For this review, take the finished solid that the model builds, in its own axes (mm). A direction names the side the tool comes from. Coordinates: 2 decimals unless noted, no trailing zeros. Write each loop counter-clockwise with the first axis right and the second up, starting at its lowest first coordinate (ties: lowest second). Pieces come first, ordered by that corner, then holes.
```python
from build123d import *

# Parameters (mm, degrees)
ESBO_O1_R                  = 12.15
RESSALTO_EXTRUS_O1_DEPTH   = 15
ESBO_O2_R                  = 4.5
RESSALTO_EXTRUS_O2_DEPTH   = 15.5
ESBO_O3_R                  = 0.9
CORTE_EXTRUS_O1_DEPTH      = 19.5
CORTE_EXTRUS_O1_DEPTH_BACK = 15.5


with BuildPart() as part:
    # Esboço1 → Ressalto-extrusão1 (new body)
    with BuildSketch(Plane.XY):
        Circle(ESBO_O1_R)
    extrude(amount=RESSALTO_EXTRUS_O1_DEPTH)

    # Esboço2 → Ressalto-extrusão2 (add)
    with BuildSketch(Plane.XY):
        Circle(ESBO_O2_R)
    extrude(amount=RESSALTO_EXTRUS_O2_DEPTH)

    # Esboço3 → Corte-extrusão1 (cut, two sides)
    with BuildSketch(Plane.XY) as corte_extrus_o1_sk:
        Circle(ESBO_O3_R)
    extrude(amount=CORTE_EXTRUS_O1_DEPTH, mode=Mode.SUBTRACT)
    extrude(corte_extrus_o1_sk.sketch, amount=-CORTE_EXTRUS_O1_DEPTH_BACK, mode=Mode.SUBTRACT)


solid = part.part
```
Q1. Tool access review of faces 1 (the flat face through (-1.1, 0.1, 15.5)), 2 (the flat face through (5, 0, 15)): name each direction out of +Z, -Z, +X, -X, +Y, -Y from which nothing blocks a thin tool from reaching the whole face with its end or side.
Ans:
face 1: +Z, +X, -X, +Y, -Y
face 2: +Z
Q2. Draft analysis for pull direction X (two halves, no side actions). For faces 3 (the cylindrical face through (0.86, 0.27, 7.64)), 4 (the cylindrical face through (-2.63, -11.86, 7.4)), 5 (the flat face through (0, -3, 0)), state which applies: +X half, -X half, draft (parallel to the pull), parting line (faces both ways), or undercut.
Ans:
face 3: undercut
face 4: parting line
face 5: draft
Q3. Add section A-A (y = 0). State the section outline as (x, z) points.
Ans:
outline: (-12.15, 0) - (-0.9, 0) - (-0.9, 15.5) - (-4.5, 15.5) - (-4.5, 15) - (-12.15, 15) - close; (0.9, 0) - (12.15, 0) - (12.15, 15) - (4.5, 15) - (4.5, 15.5) - (0.9, 15.5) - close
Q4. For probe 1 along Y at (x, z) = (0, 6.5); probe 2 along Z at (x, y) = (-2.75, -7.5); probe 3 along Y at (x, z) = (-0.75, 1), list the stretches that pass through material, from the lowest coordinate up.
Ans:
probe 1: y = -12.15 to -0.9, 0.9 to 12.15
probe 2: z = 0 to 15
probe 3: y = -12.13 to -0.5, 0.5 to 12.13
Q5. Add section C-C (z = 7.25). State the section outline as (x, y) points.
Ans:
outline: circle Ø24.3 at (0, 0); hole circle Ø1.8 at (0, 0)
Q6. Clearance check with flat-ended pins moving along their axes: pin 1 Ø3 at (x, z) = (5.5, 4) entering from +Y; pin 2 Ø5 at (y, z) = (7, 13.5) entering from -X; pin 3 Ø1 at (y, z) = (3.5, 8.5) entering from -X. State where each tip first meets the part, or that it passes through.
Ans:
pin 1: stops at y = 11.47
pin 2: stops at x = -11.29
pin 3: stops at x = -11.77
Q7. Add section D-D (x = -10.5). State the section outline as (y, z) points.
Ans:
outline: (-6.11, 0) - (6.11, 0) - (6.11, 15) - (-6.11, 15) - close
